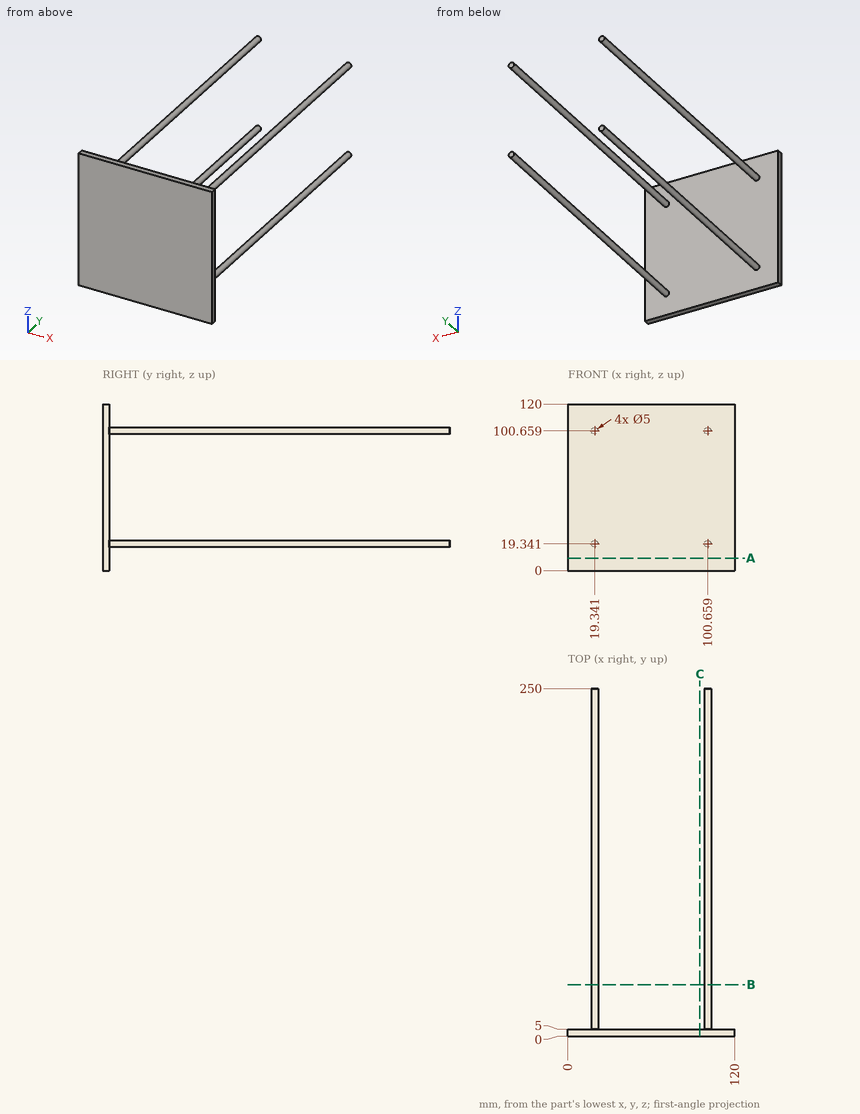
Here's the drawing with two shaded views (mm, measured from the low corner). I have some questions. Give positions to 0.01 mm unless a question says otherwise; leave off trailing zeros. Loops run counter-clockwise (first coordinate to the right, second up) from the corner with the lowest first, then second, coordinate; pieces in that order, holes last. Notation, with made-up numbers: (86.25, 46.5) - (116.25, 46.5) arc R21 ccw to (116.25, 83.5) - close; hole circle Ø1 at (-30, 0.5). An arc over 180 degrees is marked (long way). One line per item, written item: value.
(1) If we section it at C-C, the plane x = 95: List the corners of the cut face in (y, z) for me, plus the area to 3 significant figures.
Verdict:
outline: (0, 0) - (5, 0) - (5, 120) - (0, 120) - close
area: 600 mm^2
(2) If we section it at B-B, the plane y = 37: List the corners of the cut face in (x, z) for me.
Verdict:
outline: circle Ø5 at (19.34, 19.34); circle Ø5 at (19.34, 100.66); circle Ø5 at (100.66, 19.34); circle Ø5 at (100.66, 100.66)
(3) I'm going to push flat-ended pins straight in: pin 1 (5 mm diameter, centred on x = 18.5, z = 84.5, fed in from +Y); pin 2 (5 mm diameter, centred on y = 38, z = 101, fed in from -X); pin 3 (1.5 mm diameter, centred on y = 121, z = 98.5, fed in from -X) (1 decimal). Where does each tip first touch, or does it pass through?
Verdict:
pin 1: y = 5
pin 2: x = 16.84
pin 3: x = 17.3
(4) I need wall thicknesses on line 1 along X through (y, z) = (199, 19) (1 decimal); line 2 along Y through (x, z) = (93.5, 45.5). Which ranges of each line are inside material? Lowest first, please.
Verdict:
line 1: 16.9 to 21.8, 98.2 to 103.1
line 2: 0 to 5
(5) If we section it at A-A, the plane z = 9: List the corners of the cut face in (x, y) for me, plus the area to 3 significant figures.
Verdict:
outline: (0, 0) - (120, 0) - (120, 5) - (0, 5) - close
area: 600 mm^2
